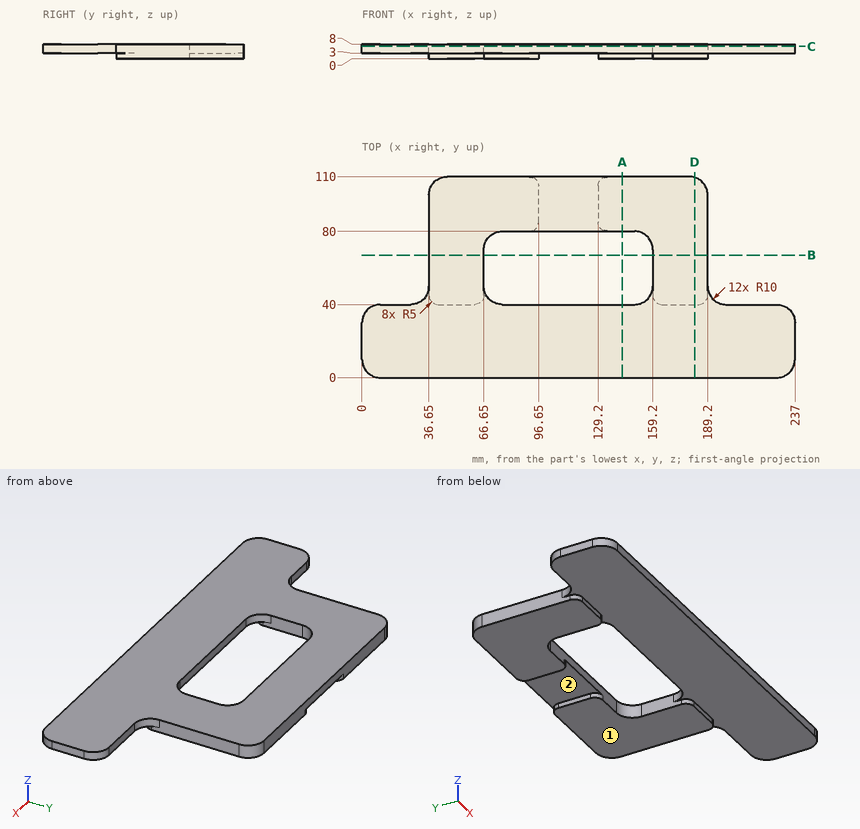
Verification items for this drawing (mm, ordinates from the low corner). Coordinates: 2 decimals unless noted, no trailing zeros. Order: outer loops, then holes, each group sorted by start corner. A loop starts at its lowest first (then second) coordinate and runs counter-clockwise, first axis right, second up. Notation, with made-up numbers: (4, 58) - (19, 58) arc R18 ccw to (19, 81) - close; hole circle Ø5 at (43.25, 80). An arc over 180 degrees is marked (long way). Answer in a Markdown table with one row per item. Add a question column.
1. Section check C-C (z = 6.75). Enter the section's corners in (x, y).
2. Section check A-A (x = 142.5). Enter the section's corners in (y, z).
3. Draft check along X on the marked faces 1 and 2. Enter one of: +X half, -X half, draft (parallel to the pull), parting line (faces both ways), or undercut.
4. Gauge pin test, flat ends, axial feed: pin 1 Ø2.5 at (x, z) = (22.5, 6) entering from +Y; pin 2 Ø1 at (y, z) = (58.5, 2) entering from +X; pin 3 Ø0.9 at (x, z) = (176.5, 1.5) entering from -Y. Record the tip position at first contact, or that the pin passes through.
5. Section check B-B (y = 67). Enter the section's corners in (x, z), plus the area to 3 significant figures.
6. Section check D-D (x = 182). Enter the section's corners in (y, z), plus the area to 3 significant figures.
7. Material ranges on L1, parallel to X at y = 65, z = 1.5; L2, parallel to Y at x = 136.5, z = 7.25; L3, parallel to X at y = 49, z = 3.25, recorded low to high. Write a range as [from, to].
Data:
| question | item | result |
|---|---|---|
| 1 | outline | (0, 10) arc R10 ccw to (10, 0) - (227, 0) arc R10 ccw to (237, 10) - (237, 30) arc R10 ccw to (227, 40) - (199.2, 40) arc R10 cw to (189.2, 50) - (189.2, 100) arc R10 ccw to (179.2, 110) - (46.65, 110) arc R10 ccw to (36.65, 100) - (36.65, 50) arc R10 cw to (26.65, 40) - (10, 40) arc R10 ccw to (0, 30) - close; hole (66.65, 50) arc R10 ccw to (76.65, 40) - (149.2, 40) arc R10 ccw to (159.2, 50) - (159.2, 70) arc R10 ccw to (149.2, 80) - (76.65, 80) arc R10 ccw to (66.65, 70) - close |
| 2 | outline | (0, 3) - (40, 3) - (40, 8) - (0, 8) - close; (80, 0) - (110, 0) - (110, 8) - (80, 8) - close |
| 3 | face 1 | draft |
| 3 | face 2 | undercut |
| 4 | pin 1 | stops at y = 40 |
| 4 | pin 2 | stops at x = 189.2 |
| 4 | pin 3 | stops at y = 40 |
| 5 | outline | (36.65, 0) - (66.65, 0) - (66.65, 8) - (36.65, 8) - close; (159.2, 0) - (189.2, 0) - (189.2, 8) - (159.2, 8) - close |
| 5 | area | 480 mm² |
| 6 | outline | (0, 3) - (40, 3) - (40, 0) - (109.6, 0) - (109.6, 8) - (0, 8) - close |
| 6 | area | 757 mm² |
| 7 | L1 | x = [36.65, 66.65], [159.2, 189.2] |
| 7 | L2 | y = [0, 40], [80, 110] |
| 7 | L3 | x = [36.6, 66.7], [159.15, 189.25] |
